Design review of the part built by this model. Coordinates are the model's own, in mm. A direction names the side the tool comes from. Coordinates: 2 decimals unless noted, no trailing zeros. Order: outer loops, then holes, each group sorted by start corner. A loop starts at its lowest first (then second) coordinate and runs counter-clockwise, first axis right, second up. Notation, with made-up numbers: M 21.5,6.5 L 42.5,6.5 A12 cw 42.5,24.5 Z; hole C 1.25,-35.75 d8. An arc over 180 degrees is marked long. Answer in a Markdown table with one row per item.
from build123d import *

# Parameters (mm, degrees)
F0_R     = 2
F1_DEPTH = 1


with BuildPart() as f1:
    # F0 (on Top) → F1 (new body)
    with BuildSketch(Plane.XY):
        Polygon((-170.931182, 94.929279), (-178.935592, 100.393385), (-174.19368, 83.114073), (-165.403008, 79.330623), (-165.294349, 77.884942), (-169.487819, 73.585391), (-178.64053, 76.696806), (-169.576123, 61.166067), (-160.313651, 59.888694), (-159.703866, 58.582332), (-162.630156, 53.304747), (-172.268271, 53.874396), (-159.703866, 41.302852), (-150.326058, 42.545263), (-149.290547, 41.406386), (-150.843814, 35.401404), (-160.297245, 33.490323), (-144.676849, 24.660785), (-135.845885, 28.173612), (-134.896323, 27.366612), (-134.896323, 21.229759), (-143.300653, 16.94699), (-126.037876, 12.481747), (-118.515134, 18.081743), (-117.21383, 17.592588), (-115.578801, 11.634614), (-122.706801, 5.295417), (-104.921646, 5.295417), (-98.986857, 12.843247), (-97.754188, 12.843247), (-94.544627, 7.404838), (-99.824868, -0.601654), (-82.638197, 4.195278), (-78.807436, 12.843247), (-77.541642, 13.009544), (-73.138356, 8.775612), (-76.111726, -0.265788), (-60.774289, 8.775612), (-59.456516, 18.109852), (-58.175348, 18.658925), (-52.757829, 15.657326), (-53.416714, 6.030248), (-40.861767, 18.76732), (-41.971847, 28.13928), (-40.861767, 29.065885), (-34.913585, 27.52826), (-32.994203, 18.100707), (-24.199748, 33.567108), (-27.712576, 42.396642), (-26.905576, 43.499492), (-20.779634, 43.600194), (-16.44348, 35.033159), (-11.998242, 52.313395), (-17.667146, 59.771266), (-17.104328, 61.170273), (-11.314055, 62.781483), (-4.805986, 55.59827), (-4.969601, 73.500365), (-12.407549, 79.304725), (-12.317293, 80.623472), (-7.000638, 83.757633), (1.064408, 78.466788), (-3.74119, 95.745668), (-12.317293, 99.474117), (-12.467637, 100.935459), (-8.347162, 105.220751), (0.74094, 102.232022), (-8.272784, 117.522509), (-17.522758, 118.920013), (-18.108435, 120.23779), (-15.069733, 125.581815), (-5.598881, 124.933623), (-18.290413, 137.443681), (-27.662303, 136.307329), (-28.557425, 137.438729), (-27.033923, 143.36113), (-17.676375, 145.266259), (-33.176269, 154.079758), (-41.853711, 150.553182), (-43.134663, 151.459798), (-43.134663, 157.608002), (-34.616161, 161.854208), (-51.867886, 166.292111), (-59.378833, 160.689354), (-60.774289, 161.31033), (-62.388756, 167.115263), (-55.173125, 173.475817), (-72.983663, 173.313039), (-78.776218, 165.940508), (-80.316429, 166.045921), (-83.425997, 171.320856), (-77.970915, 179.398346), (-95.370838, 174.559084), (-98.986857, 165.907577), (-100.430792, 165.759024), (-104.825104, 169.984327), (-101.852417, 179.02365), (-117.040908, 170.070053), (-118.387379, 160.870731), (-119.778854, 160.177124), (-125.139098, 163.225048), (-124.489884, 172.71082), (-137.053189, 159.965269), (-135.889679, 150.703996), (-137.053189, 149.78347), (-142.977322, 151.307418), (-144.888788, 160.696093), (-153.754356, 145.104628), (-150.389701, 136.644378), (-151.345882, 135.293397), (-157.080024, 135.293397), (-161.457264, 144.074773), (-165.973303, 126.519309), (-160.271138, 118.921481), (-160.782874, 117.619239), (-166.658001, 115.98525), (-173.070462, 123.259766), (-173.070462, 105.623409), (-165.534943, 99.514894), (-165.635112, 98.051306), align=None)
        with Locations((-89.083396, 89.265883)):
            Circle(F0_R, mode=Mode.SUBTRACT)
    extrude(amount=F1_DEPTH)


solid = f1.part
(1) For line 1 along Y through (x, z) = (-168, 0.4); line 2 along Y through (x, z) = (-166.5, 0.1); line 3 along Y through (x, z) = (-90.5, 0.9), list the stretches that pass through material, from the lowest coordinate up. Write a range as from..to.
Return value:
| item | result |
|---|---|
| line 1 | y = 49.6..53.62, 60.95..75.11, 80.45..96.66, 101.51..117.51 |
| line 2 | y = 48.1..53.53, 60.74..76.65, 79.8..97.54, 100.3..116.03 |
| line 3 | y = 2..87.85, 90.68..175.91 |
(2) Insertion check: pin 1 Ø0.5 at (x, z) = (-153.5, 0.5) entering from +Y; pin 2 Ø0.5 at (y, z) = (155.5, 0.5) entering from +X. Each pin has a flat end and moves straight along its axis. Give the tip position at first contact, or say it passes through.
Return value:
| item | result |
|---|---|
| pin 1 | stops at y = 145.99 |
| pin 2 | stops at x = -43.13 |
(3) Add section B-B, the plane y = 108.5. Give the boundary of the cut face in (x, z).
Return value:
| item | result |
|---|---|
| outline | M -173.07,0 L -2.95,0 L -2.95,1 L -173.07,1 Z |
(4) Draft analysis for pull direction X (two halves, no side actions). For faces 4 (the cylindrical face through (-87.176, 89.867, 0.493)), 5 (the flat face through (-3.703, 109.77, 0.493)), 6 (the flat face through (-90, 71, 1)), 7 (the flat face through (-167.362, 75.765, 0.493)), state which applies: pulls with the +X half, pulls with the -X half, needs draft (parallel to the pull), parting line crosses it, or undercut.
Return value:
| item | result |
|---|---|
| face 4 | undercut |
| face 5 | pulls with the +X half |
| face 6 | needs draft |
| face 7 | undercut |
(5) Add section A-A, the plane x = -128.5. Give the boundary of the cut face in (y, z).
Return value:
| item | result |
|---|---|
| outline | M 13.12,0 L 168.64,0 L 168.64,1 L 13.12,1 Z |
(6) For faces 1 (the flat face through (-109.34, 174.61, 0.49)), 2 (the flat face through (-38.94, 159.7, 0.49)), 3 (the flat face through (-14.8, 56, 0.5)), list the 3-axis set-ups (+Z, -Z, +X, -X, +Y, -Y) from which the entire face can be reached by the end or side of a thin tool; tool diameter is ignored.
Return value:
| item | result |
|---|---|
| face 1 | +Z, -Z, +Y |
| face 2 | +Z, -Z, +X |
| face 3 | +Z, -Z |
